from build123d import *

# Parameters (mm, degrees)
SKETCH1_R           = 3
BOSS_EXTRUDE1_DEPTH = 10
SKETCH2_W           = 10
SKETCH2_H           = 5
BOSS_EXTRUDE2_DEPTH = 2
SKETCH3_W           = 10
SKETCH3_H           = 1
CUT_EXTRUDE1_DEPTH  = 1


with BuildPart() as part:
    # Sketch1 → Boss-Extrude1 (new body)
    with BuildSketch(Plane(origin=(0, 0, 0), x_dir=(1, 0, 0), z_dir=(0, 1, 0))):
        with Locations(Location((0, 0, 0), (0, 0, 270))):
            Circle(SKETCH1_R)
    extrude(amount=BOSS_EXTRUDE1_DEPTH)

    # Sketch2 → Boss-Extrude2 (add)
    with BuildSketch(Plane(origin=(0, 10, 0), x_dir=(1, 0, 0), z_dir=(0, 1, 0))):
        Rectangle(SKETCH2_W, SKETCH2_H)
    extrude(amount=BOSS_EXTRUDE2_DEPTH)

    # Sketch3 → Cut-Extrude1 (cut)
    with BuildSketch(Plane(origin=(0, 12, 0), x_dir=(1, 0, 0), z_dir=(0, 1, 0))):
        Rectangle(SKETCH3_W, SKETCH3_H)
    extrude(amount=-CUT_EXTRUDE1_DEPTH, mode=Mode.SUBTRACT)


solid = part.part
The model under review builds one solid part; all positions refer to its coordinate system, in mm. A direction names the side the tool comes from. Coordinates: 2 decimals unless noted, no trailing zeros. Order: outer loops, then holes, each group sorted by start corner. A loop starts at its lowest first (then second) coordinate and runs counter-clockwise, first axis right, second up. Notation, with made-up numbers: (-38.5, 23) -> (-22.5, 23) arc R16 ccw to (-22.5, 42) -> close; hole circle Ø5 at (16.5, -10.5). An arc over 180 degrees is marked (long way). Answer in a Markdown table with one row per item.
(1) The part is to be moulded in two halves that separate along Z. For faces 1 (the flat face through (-5, 10.8, 0)), 2 (the flat face through (-0.1, 11.5, -0.5)), 3 (the flat face through (0, 11, -2.5)), say which applies: +Z half, -Z half, draft (parallel to the pull), parting line (faces both ways), or undercut.
Answers:
| item | result |
|---|---|
| face 1 | draft |
| face 2 | undercut |
| face 3 | -Z half |
(2) Consider section C-C (y = 7.75). Write out the cut boundary in (x, z).
Answers:
| item | result |
|---|---|
| outline | circle Ø6 at (0, 0) |
(3) Insertion check: pin 1 (1 mm diameter, centred on x = 3.5, z = 0.5, fed in from -Y); pin 2 (6 mm diameter, centred on x = 3.5, y = 10, fed in from +Z); pin 3 (1.5 mm diameter, centred on x = 3.5, y = 6, fed in from +Z). Each pin has a flat end and moves straight along its axis. Give the tip position at first contact, or say it passes through.
Answers:
| item | result |
|---|---|
| pin 1 | y = 10 |
| pin 2 | z = 2.96 |
| pin 3 | z = 1.2 |
(4) Consider section A-A (z = 0). Write out the cut boundary in (x, y), plus the area to 3 significant figures.
Answers:
| item | result |
|---|---|
| outline | (-5, 10) -> (-3, 10) -> (-3, 0) -> (3, 0) -> (3, 10) -> (5, 10) -> (5, 11) -> (-5, 11) -> close |
| area | 70.0 mm² |
(5) Consider section D-D (x = 4). Write out the cut boundary in (y, z).
Answers:
| item | result |
|---|---|
| outline | (10, -2.5) -> (12, -2.5) -> (12, -0.5) -> (11, -0.5) -> (11, 0.5) -> (12, 0.5) -> (12, 2.5) -> (10, 2.5) -> close |
(6) Machinability: for faces 4 (the cylindrical face through (0.9, 4.93, 2.86)), 5 (the flat face through (0, 11, 2.5)), 6 (the flat face through (-0.1, 11.5, 0.5)), which of the approach directions +Z, -Z, +X, -X, +Y, -Y give a long, thin tool a straight path to every point of the face, cutting with its end or side? Answer none if there is none.
Answers:
| item | result |
|---|---|
| face 4 | -Y |
| face 5 | +Z, +X, -X, +Y |
| face 6 | +X, -X, +Y |
(7) Wall thickness on line 1 along Y through (x, z) = (4.25, -0.6); line 2 along Z through (x, y) = (-2.5, 1.5); line 3 along Y through (x, z) = (1.5, -0.35): over which ranges is each line inside the solid? List them lowest first.
Answers:
| item | result |
|---|---|
| line 1 | 10 to 12 |
| line 2 | -1.66 to 1.66 |
| line 3 | 0 to 11 |
(8) Consider section B-B (x = 2.5). Write out the cut boundary in (y, z).
Answers:
| item | result |
|---|---|
| outline | (0, -1.66) -> (10, -1.66) -> (10, -2.5) -> (12, -2.5) -> (12, -0.5) -> (11, -0.5) -> (11, 0.5) -> (12, 0.5) -> (12, 2.5) -> (10, 2.5) -> (10, 1.66) -> (0, 1.66) -> close |
